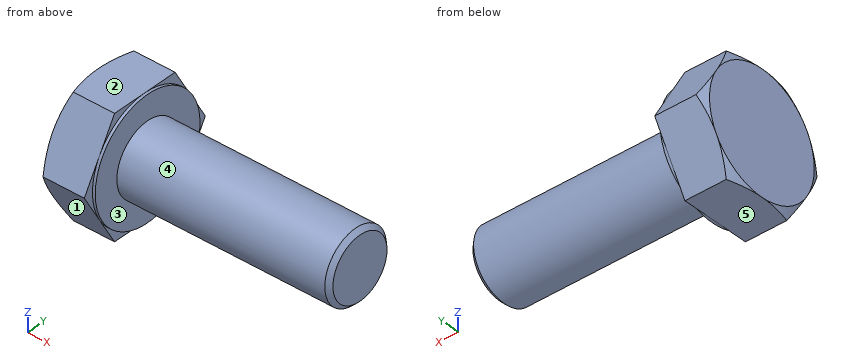
```python
from build123d import *

# Parameters (mm, degrees)
EXTRUDE_559_DEPTH = 6.6
CHAMFER_2_SIZE    = 0.61345
CHAMFER_2_SIZE2   = 0.61355


with BuildPart() as part:
    # 草圖1 → Revolve 409 (revolve)
    with BuildSketch(Plane.XY):
        Polygon((-0.4001, 0), (30, 0), (30, 5), (3, 5), (2.38645, 5), (0, 5), (0, 8.5), (-0.4001, 8.5), align=None)
    revolve(axis=Axis((30, 0, 0), (-1, 0, 0)))

    # 草圖2 → Extrude 559 (add)
    with BuildSketch(Plane.ZY.offset(0.4001)):
        Polygon((0, 9.814954576), (8.5, 4.907477288), (8.5, -4.907477288), (0, -9.814954576), (-8.5, -4.907477288), (-8.5, 4.907477288), align=None)
    extrude(amount=EXTRUDE_559_DEPTH)

    # 草圖3 → Cut-Revolve 678 (revolve, cut)
    with BuildSketch(Plane.XY):
        Polygon((-7.0001, 8.5), (-7.0001, 9.814954576), (-6.240910621, 9.814954576), align=None)
    revolve(axis=Axis((-8.3201, 0, 0), (1, 0, 0)), mode=Mode.SUBTRACT)

    # 倒角2
    chamfer_2_edges = [part.edges().sort_by_distance(p)[0] for p in [
        (30, -5, 0),
    ]]
    chamfer_2_side = [part.faces().sort_by_distance(p)[0] for p in [
        (30, 0, 0),
    ]]
    chamfer(chamfer_2_edges, length=CHAMFER_2_SIZE, length2=CHAMFER_2_SIZE2, reference=chamfer_2_side[0])


solid = part.part
```
For this review, take the finished solid that the model builds, in its own axes (mm). Face numbers are marked on the shaded views. A direction names the side the tool comes from. Round coordinates to 2 decimals unless told otherwise and drop trailing zeros. Order: outer loops, then holes, each group sorted by start corner. A loop starts at its lowest first (then second) coordinate and runs counter-clockwise, first axis right, second up.
Q1. We need section A-A, the plane x = 19. Give the boundary of the cut face in (y, z).
Findings below:
outline: circle Ø10 at (0, 0)
Q2. Machinability: for the marked faces 4 and 5, which of the approach directions +Z, -Z, +X, -X, +Y, -Y give a long, thin tool a straight path to every point of the face, cutting with its end or side? Answer none if there is none.
Findings below:
face 4: +X
face 5: -Z, +X, -X, +Y, -Y
Q3. Insertion check: P1, Ø1.2, axis at y = -8.5, z = 0.5, coming from the +X side; P2, Ø2, axis at x = 11, z = 5, coming from the -Y side; P3, Ø1, axis at x = -2, z = -4, coming from the -Y side. Each pin has a flat end and moves straight along its axis. Give the tip position at first contact, or say it passes through.
Findings below:
P1: stops at x = 0
P2: stops at y = -3
P3: stops at y = -7.79
Q4. Wall thickness on line 1 (X direction, y = 5.75, z = 5.5); line 2 (Y direction, x = 11, z = 0); line 3 (Y direction, x = -2, z = 8.25): over which ranges is each line inside the solid? List them lowest first.
Findings below:
line 1: x = -7 to 0
line 2: y = -5 to 5
line 3: y = -5.05 to 5.05
Q5. Mouldability with a two-part tool opening along Z and no side actions: class the marked faces 1, 2 and 3 as pulls with the +Z half, pulls with the -Z half, needs draft (parallel to the pull), parting line crosses it, or undercut.
Findings below:
face 1: pulls with the -Z half
face 2: pulls with the +Z half
face 3: needs draft
